```python
from build123d import *

# Parameters (mm, degrees)
Y_KSEKLIK_EKSTR_ZYON1_DEPTH = 9
Y_KSEKLIK_EKSTR_ZYON2_DEPTH = 6
IZIM4_R                     = 1.5
IZIM4_R_2                   = 2.5
KES_EKSTR_ZYON2_DEPTH       = 6.5
IZIM5_W                     = 14
IZIM5_H                     = 15
Y_KSEKLIK_EKSTR_ZYON3_DEPTH = 5
Y_KSEKLIK_EKSTR_ZYON4_DEPTH = 7
IZIM3_W                     = 7.2
IZIM3_H                     = 2
IZIM3_W_2                   = 2
IZIM3_H_2                   = 8.3
KES_EKSTR_ZYON3_DEPTH       = 3
IZIM8_R                     = 1.5
KES_EKSTR_ZYON5_DEPTH       = 10
IZIM9_R                     = 2.5
IZIM9_R_2                   = 4
KES_EKSTR_ZYON6_DEPTH       = 2
IZIM10_R                    = 2.5
KES_EKSTR_ZYON7_DEPTH       = 2
KES_EKSTR_ZYON8_START       = -10
KES_EKSTR_ZYON8_DEPTH       = 10
IZIM12_W                    = 14
IZIM12_H                    = 3
Y_KSEKLIK_EKSTR_ZYON5_DEPTH = 5


with BuildPart() as part:
    # izim1 → Y_kseklik-Ekstr_zyon1 (new body)
    with BuildSketch(Plane.XY):
        with BuildLine():
            Line((17, 7), (17, -7))
            ThreePointArc((17, -7), (14.071067812, -14.071067812), (7, -17))
            Line((7, -17), (-7, -17))
            ThreePointArc((-7, -17), (-14.071067812, -14.071067812), (-17, -7))
            Line((-17, -7), (-17, 7))
            ThreePointArc((-17, 7), (-14.071067812, 14.071067812), (-7, 17))
            Line((-7, 17), (7, 17))
            ThreePointArc((7, 17), (14.071067812, 14.071067812), (17, 7))
        make_face()
        with BuildLine():
            Line((-7, 12), (7, 12))
            ThreePointArc((7, 12), (10.535533906, 10.535533906), (12, 7))
            Line((12, 7), (12, -7))
            ThreePointArc((12, -7), (10.535533906, -10.535533906), (7, -12))
            Line((7, -12), (-7, -12))
            ThreePointArc((-7, -12), (-10.535533906, -10.535533906), (-12, -7))
            Line((-12, -7), (-12, 7))
            ThreePointArc((-12, 7), (-10.535533906, 10.535533906), (-7, 12))
        make_face(mode=Mode.SUBTRACT)
    extrude(amount=Y_KSEKLIK_EKSTR_ZYON1_DEPTH)

    # izim2 → Y_kseklik-Ekstr_zyon2 (add)
    with BuildSketch(Plane.XY):
        with BuildLine():
            Line((-7, -12), (7, -12))
            ThreePointArc((7, -12), (10.535533906, -10.535533906), (12, -7))
            Line((12, -7), (12, 7))
            ThreePointArc((12, 7), (10.535533906, 10.535533906), (7, 12))
            Line((7, 12), (-7, 12))
            ThreePointArc((-7, 12), (-10.535533906, 10.535533906), (-12, 7))
            Line((-12, 7), (-12, -7))
            ThreePointArc((-12, -7), (-10.535533906, -10.535533906), (-7, -12))
        make_face()
    extrude(amount=Y_KSEKLIK_EKSTR_ZYON2_DEPTH)

    # izim4 → Kes-Ekstr_zyon2 (cut)
    with BuildSketch(Plane.XY.offset(6)):
        with Locations((0, 9)):
            Circle(IZIM4_R)
        Circle(IZIM4_R_2)
        with Locations((9, 0)):
            Circle(IZIM4_R)
        with Locations((0, -9)):
            Circle(IZIM4_R)
        with Locations((-9, 0)):
            Circle(IZIM4_R)
    extrude(amount=-KES_EKSTR_ZYON2_DEPTH, mode=Mode.SUBTRACT)

    # izim5 → Y_kseklik-Ekstr_zyon3 (add)
    with BuildSketch(Plane.XY):
        with Locations((0, -24.5)):
            Rectangle(IZIM5_W, IZIM5_H)
    extrude(amount=Y_KSEKLIK_EKSTR_ZYON3_DEPTH)

    # izim6 → Y_kseklik-Ekstr_zyon4 (add, symmetric)
    with BuildSketch(Plane(origin=(0, 0, 0), x_dir=(0, 0, -1), z_dir=(1, 0, 0))):
        with BuildLine():
            Line((0, -32), (-5, -32))
            Line((-5, -32), (-5, -57))
            ThreePointArc((-5, -57), (-10, -62), (-15, -57))
            Line((-15, -57), (-15, -47))
            Line((-15, -47), (-20, -47))
            Line((-20, -47), (-20, -57))
            ThreePointArc((-20, -57), (-10, -67), (0, -57))
            Line((0, -57), (0, -32))
        make_face()
    extrude(amount=Y_KSEKLIK_EKSTR_ZYON4_DEPTH, both=True)

    # izim3 → Kes-Ekstr_zyon3 (cut)
    with BuildSketch(Plane.XY.offset(6)):
        with Locations((8.4, 2.7)):
            Rectangle(IZIM3_W, IZIM3_H)
        with Locations((2.7, 7.85)):
            Rectangle(IZIM3_W_2, IZIM3_H_2)
        with Locations((-2.7, 7.85)):
            Rectangle(IZIM3_W_2, IZIM3_H_2)
        with Locations((-8.4, 2.7)):
            Rectangle(IZIM3_W, IZIM3_H)
        with Locations((-8.4, -2.7)):
            Rectangle(IZIM3_W, IZIM3_H)
        with Locations((-2.7, -7.85)):
            Rectangle(IZIM3_W_2, IZIM3_H_2)
        with Locations((2.7, -7.85)):
            Rectangle(IZIM3_W_2, IZIM3_H_2)
        with Locations((8.4, -2.7)):
            Rectangle(IZIM3_W, IZIM3_H)
    extrude(amount=-KES_EKSTR_ZYON3_DEPTH, mode=Mode.SUBTRACT)

    # izim8 → Kes-Ekstr_zyon5 (cut)
    with BuildSketch(Plane.XY.offset(20)):
        with Locations((-4, -51.616632033)):
            Circle(IZIM8_R)
        with Locations((4, -51.616632033)):
            Circle(IZIM8_R)
    extrude(amount=-KES_EKSTR_ZYON5_DEPTH, mode=Mode.SUBTRACT)

    # izim9 → Kes-Ekstr_zyon6 (cut)
    with BuildSketch(Plane(origin=(0, 0, 0), x_dir=(-1, 0, 0), z_dir=(0, 0, -1))):
        with Locations((0, 9)):
            Circle(IZIM9_R)
        Circle(IZIM9_R_2)
        with Locations((9, 0)):
            Circle(IZIM9_R)
        with Locations((0, -9)):
            Circle(IZIM9_R)
        with Locations((-9, 0)):
            Circle(IZIM9_R)
    extrude(amount=-KES_EKSTR_ZYON6_DEPTH, mode=Mode.SUBTRACT)

    # izim10 → Kes-Ekstr_zyon7 (cut)
    with BuildSketch(Plane.XY.offset(20)):
        with Locations((-4, -51.616632033)):
            Circle(IZIM10_R)
        with Locations((4, -51.616632033)):
            Circle(IZIM10_R)
    extrude(amount=-KES_EKSTR_ZYON7_DEPTH, mode=Mode.SUBTRACT)

    # izim11 → Kes-Ekstr_zyon8 (cut)
    with BuildSketch(Plane.XY.offset(9).offset(KES_EKSTR_ZYON8_START)):
        with BuildLine():
            Line((7, 17), (-7, 17))
            ThreePointArc((-7, 17), (-14.071067812, 14.071067812), (-17, 7))
            Line((-17, 7), (-17, -7))
            ThreePointArc((-17, -7), (-14.071067812, -14.071067812), (-7, -17))
            Line((-7, -17), (7, -17))
            ThreePointArc((7, -17), (14.071067812, -14.071067812), (17, -7))
            Line((17, -7), (17, 7))
            ThreePointArc((17, 7), (14.071067812, 14.071067812), (7, 17))
        make_face()
        with BuildLine():
            Line((7, 14), (-7, 14))
            ThreePointArc((-7, 14), (-11.949747468, 11.949747468), (-14, 7))
            Line((-14, 7), (-14, -7))
            ThreePointArc((-14, -7), (-11.949747468, -11.949747468), (-7, -14))
            Line((-7, -14), (7, -14))
            ThreePointArc((7, -14), (11.949747468, -11.949747468), (14, -7))
            Line((14, -7), (14, 7))
            ThreePointArc((14, 7), (11.949747468, 11.949747468), (7, 14))
        make_face(mode=Mode.SUBTRACT)
    extrude(amount=KES_EKSTR_ZYON8_DEPTH, mode=Mode.SUBTRACT)


with BuildPart() as kes_ekstr_zyon8_piece_1:
    # of the separate pieces the step leaves, piece 1, a body of its own (kes_ekstr_zyon8_pieces)
    add(part.part.solids().sort_by_distance((-7, -57, 0))[0])



with BuildPart() as kes_ekstr_zyon8_piece_2:
    # of the separate pieces the step leaves, piece 2, a body of its own (kes_ekstr_zyon8_pieces)
    add(part.part.solids().sort_by_distance((7, 14, 0))[0])


with BuildPart() as kes_ekstr_zyon8_piece_1_1:
    add(kes_ekstr_zyon8_piece_1.part)

    add(kes_ekstr_zyon8_piece_2.part)  # Y_kseklik-Ekstr_zyon5 merges Kes-Ekstr_zyon8 piece 2
    # izim12 → Y_kseklik-Ekstr_zyon5 (add)
    with BuildSketch(Plane.XY):
        with Locations((0, -15.5)):
            Rectangle(IZIM12_W, IZIM12_H)
    extrude(amount=Y_KSEKLIK_EKSTR_ZYON5_DEPTH)


solid = kes_ekstr_zyon8_piece_1_1.part
```
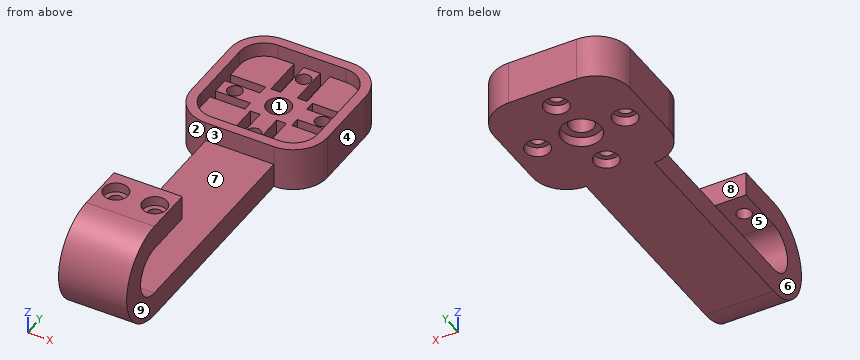
Read the model definition and answer for the solid it produces. Units are mm, in the model's axes. Face numbers are marked on the shaded views. A direction names the side the tool comes from. Coordinates: 2 decimals unless noted, no trailing zeros. Write each loop counter-clockwise with the first axis right and the second up, starting at its lowest first coordinate (ties: lowest second). Pieces come first, ordered by that corner, then holes. Notation, with made-up numbers: (-17, 39.25) -> (-13, 39.25) arc R26 cw to (-13, 66.25) -> close; hole circle Ø2 at (79.25, 75.5). An arc over 180 degrees is marked (long way). Answer as a JSON object with one key per item and string values.
Q1. Flat-ended cylindrical pins translate along their axes: pin 1 Ø3 at (x, z) = (6.5, 6.5) entering from -Y; pin 2 Ø1 at (x, y) = (3, 6.5) entering from +Z; pin 3 Ø2.5 at (x, y) = (9.5, -0.5) entering from -Z. Find the tip coordinate at first contact, or state that the pin passes through.
The answers:
{"pin 1": "stops at y = -66.8", "pin 2": "stops at z = 3", "pin 3": "stops at z = 2"}
Q2. The part is cut by section B-B on z = 6.75. Give the vertices of the cut face in (x, y).
The answers:
{"outline": "(-14, -7) arc R7 ccw to (-7, -14) -> (7, -14) arc R7 ccw to (14, -7) -> (14, 7) arc R7 ccw to (7, 14) -> (-7, 14) arc R7 ccw to (-14, 7) -> close; (-7, -66.46) -> (7, -66.46) -> (7, -60.8) -> (-7, -60.8) -> close; hole (-12, -7) arc R5 ccw to (-7, -12) -> (7, -12) arc R5 ccw to (12, -7) -> (12, 7) arc R5 ccw to (7, 12) -> (-7, 12) arc R5 ccw to (-12, 7) -> close"}
Q3. The part is cut by section C-C on y = -9. Give the vertices of the cut face in (x, z), then the cut area to 3 significant figures.
The answers:
{"outline": "(-13.71, 0) -> (-2.5, 0) -> (-2.5, 2) -> (-1.5, 2) -> (-1.5, 6) -> (-1.7, 6) -> (-1.7, 3) -> (-3.7, 3) -> (-3.7, 6) -> (-11.58, 6) -> (-11.58, 9) -> (-13.71, 9) -> close; (1.5, 2) -> (2.5, 2) -> (2.5, 0) -> (13.71, 0) -> (13.71, 9) -> (11.58, 9) -> (11.58, 6) -> (3.7, 6) -> (3.7, 3) -> (1.7, 3) -> (1.7, 6) -> (1.5, 6) -> close", "area": "143 mm2"}
Q4. Consider line 1 (X direction, y = 6, z = 4.5); line 2 (Y direction, x = 0, z = 0.9); line 3 (Y direction, x = 0, z = 4.35). Determine where each line is inside the solid, lowest interval first. Write a range as [from, to].
The answers:
{"line 1": "x = [-14, -3.7], [-1.7, 1.7], [3.7, 14]", "line 2": "y = [-61.15, -11.5], [-6.5, -4], [4, 6.5], [11.5, 14]", "line 3": "y = [-65.25, -10.5], [-7.5, -2.5], [2.5, 7.5], [10.5, 14]"}
Q5. A tool of negligible diameter and unlimited length cuts with its end or side. For the marked faces 5, 6, 7, 8 and 9, from which of +Z, -Z, +X, -X, +Y, -Y can it reach the whole face along a straight path? Write none if from no direction.
The answers:
{"face 5": "+X, -X, +Y", "face 6": "+Z, -Z, -X, -Y", "face 7": "+X, -X", "face 8": "+Z, +X, -X, +Y", "face 9": "+Z, -Z, +X, -Y"}
Q6. The part is cut by section A-A on y = 0. Give the number of separate pieces and of enclosed holes in the cut face, then the cut area to 3 significant figures.
The answers:
{"separate pieces": "4", "enclosed holes": "0", "area": "100 mm2"}
Q7. Determine the mould class of the marked faces 1, 2, 3 and 4 for opening direction Y: pulls with the +Y half, pulls with the -Y half, needs draft (parallel to the pull), parting line crosses it, or undercut.
The answers:
{"face 1": "undercut", "face 2": "pulls with the -Y half", "face 3": "undercut", "face 4": "needs draft"}
